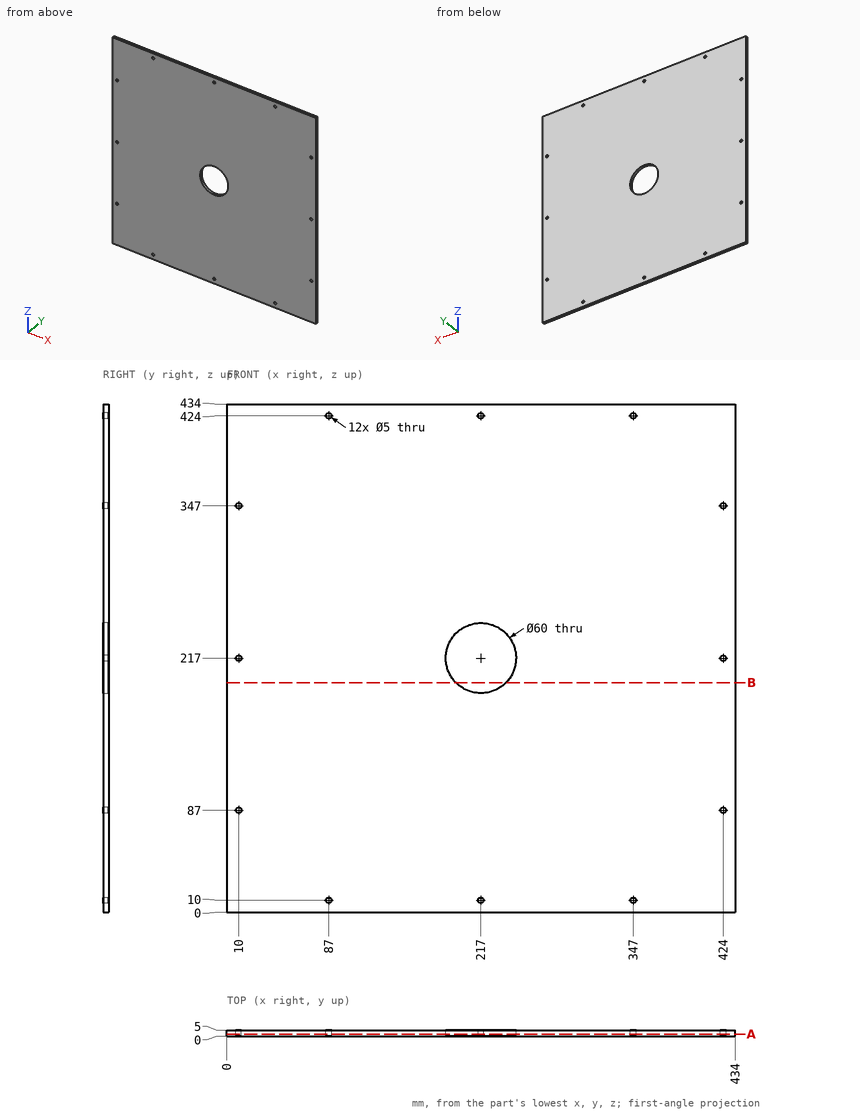
Geometry check sheet. Reference: drawing and pictorial views, mm from the part's lowest x, y, z. Coordinates: 2 decimals unless noted, no trailing zeros. Order: outer loops, then holes, each group sorted by start corner. A loop starts at its lowest first (then second) coordinate and runs counter-clockwise, first axis right, second up. Notation, with made-up numbers: M -8.75,27 L 12.25,27 A18 cw 12.25,52 Z; hole C -18,4 d7. An arc over 180 degrees is marked long. Return JSON: item names as keys, results as strings.
1) Gauge pin test, flat end, axial feed: pin 1 (4.5 mm diameter, centred on x = 217, z = 424, fed in from -Y). Record the tip position at first contact, or that the pin passes through.
Answer list:
{"pin 1": "through"}
2) Thickness scan on L1, parallel to X at y = 1.1, z = 217; L2, parallel to Z at x = 424, y = 1.5; L3, parallel to Z at x = 346.5, y = 0.7. Record the ranges inside material, lowest first. Write a range as [from, to].
Answer list:
{"L1": "[0, 7.5], [12.5, 187], [247, 421.5], [426.5, 434]", "L2": "[0, 84.5], [89.5, 214.5], [219.5, 344.5], [349.5, 434]", "L3": "[0, 7.55], [12.45, 421.55], [426.45, 434]"}
3) Cross-section at B-B, the plane z = 196. Record the boundary of the cut face in (x, y).
Answer list:
{"outline": "M 0,0 L 195.58,0 L 195.58,5 L 0,5 Z; M 238.42,0 L 434,0 L 434,5 L 238.42,5 Z"}
4) Cross-section at A-A, the plane y = 1.65. Count the separate pieces of the cut face and the enclosed holes in it, and give its area (3 significant figures).
Answer list:
{"separate pieces": "1", "enclosed holes": "13", "area": "185,000 mm2"}
